For this review, take the finished solid that the model builds, in its own axes (mm). A direction names the side the tool comes from. Round coordinates to 2 decimals unless told otherwise and drop trailing zeros. Write each loop counter-clockwise with the first axis right and the second up, starting at its lowest first coordinate (ties: lowest second). Pieces come first, ordered by that corner, then holes. Notation, with made-up numbers: M 26.5,70.25 L 81.5,70.25 A15 ccw 81.5,97.25 Z; hole C -1,57 d7. An arc over 180 degrees is marked long. One line per question, with ' | ' between items.
```python
from build123d import *

# Parameters (mm, degrees)
F1_DEPTH = 7.62
F2_R     = 12.7
F3_DEPTH = 63.5
F4_R     = 8.89
F5_DEPTH = 71.121
F6_R     = 6.35
F7_DEPTH = 57.15


with BuildPart() as f1:
    # F0 (on Top) → F1 (new body)
    with BuildSketch(Plane.XY):
        Polygon((-57.15, 50.472703), (0, -48.514001), (57.15, 50.472703), align=None)
    extrude(amount=F1_DEPTH)

    # F2 (on face) → F3 (join)
    with BuildSketch(Plane.XY.offset(7.62)):
        with Locations((0, 14.985999)):
            Circle(F2_R)
    extrude(amount=F3_DEPTH)

    # F4 (on Top) → F5 (cut, through all)
    with BuildSketch(Plane.XY):
        with Locations((0, 14.985999)):
            Circle(F4_R)
    extrude(amount=F5_DEPTH, mode=Mode.SUBTRACT)

    # F6 (on Top) → F7 (join)
    with BuildSketch(Plane.XY):
        with Locations((0, -48.499294)):
            Circle(F6_R)
        with Locations((-57.143047, 50.380189)):
            Circle(F6_R)
        with Locations((57.150319, 50.4466)):
            Circle(F6_R)
    extrude(amount=F7_DEPTH)


solid = f1.part
```
Item 1: Take a section at A-A (x = 0). Write out the cut boundary in (y, z), then the cut area to 3 significant figures.
Results:
outline: M -54.85,0 L 6.1,0 L 6.1,71.12 L 2.29,71.12 L 2.29,7.62 L -42.15,7.62 L -42.15,57.15 L -54.85,57.15 Z; M 23.88,0 L 50.47,0 L 50.47,7.62 L 27.69,7.62 L 27.69,71.12 L 23.88,71.12 Z | area: 1,780 mm2
Item 2: To check wall thickness, follow line 1 along Y through (x, z) = (0, 44.5); line 2 along Z through (x, y) = (-30.5, 9); line 3 along X through (y, z) = (9.5, 58.5). State the ranges of each line that lie inside material, in increasing order. Write a range as from..to.
Results:
line 1: -54.85..-42.15, 2.29..6.1, 23.88..27.69 | line 2: 0..7.62 | line 3: -11.45..-7, 7..11.45
Item 3: Take a section at B-B (z = 46). Write out the cut boundary in (x, y), then the cut area to 3 significant figures.
Results:
outline: C -57.14,50.38 d12.7; C 0,14.99 d25.4; C 0,-48.5 d12.7; C 57.15,50.45 d12.7; hole C 0,14.99 d17.78 | area: 638 mm2
Item 4: Insertion check: pin 1 Ø10 at (y, z) = (4, 21.5) entering from +X; pin 2 Ø1.5 at (x, z) = (20, 8.5) entering from +Y; pin 3 Ø6.5 at (x, y) = (-59, 52) entering from +Z; pin 4 Ø6 at (x, z) = (-11, 38) entering from -Y. Each pin has a flat end and moves straight along its axis. Give the tip position at first contact, or say it passes through.
Results:
pin 1: x = 11.2 | pin 2: through | pin 3: z = 57.15 | pin 4: y = 5.12
Item 5: Take a section at C-C (x = -45.5). Write out the cut boundary in (y, z).
Results:
outline: M 30.29,0 L 50.47,0 L 50.47,7.62 L 30.29,7.62 Z
Item 6: Machinability: for faces 1 (the face through (-2.8, 2.6, 38.9)), 2 (the face through (1, 50.473, 4)), 3 (the face through (0, -48, 57.15)), which of the approach directions +Z, -Z, +X, -X, +Y, -Y give a long, thin tool a straight path to every point of the face, cutting with its end or side? Answer none if there is none.
Results:
face 1: +Z | face 2: +Z, -Z, +Y | face 3: +Z, +X, -X, -Y
Item 7: Mouldability with a two-part tool opening along X and no side actions: class faces 4 (the face through (2.93, -54.133, 28.175)), 5 (the face through (-1.9, 6.3, 35.1)), 6 (the face through (-9, 12, 71.12)) as +X half, -X half, draft (parallel to the pull), parting line (faces both ways), or undercut.
Results:
face 4: parting line | face 5: undercut | face 6: draft
Item 8: Take a section at D-D (y = -2.5). Write out the cut boundary in (x, z).
Results:
outline: M -26.57,0 L 26.57,0 L 26.57,7.62 L -26.57,7.62 Z
